Read the model definition and answer for the solid it produces. Units are mm, in the model's axes. Coordinates: 2 decimals unless noted, no trailing zeros. Order: outer loops, then holes, each group sorted by start corner. A loop starts at its lowest first (then second) coordinate and runs counter-clockwise, first axis right, second up. Notation, with made-up numbers: (45, -12.5) -> (62, -12.5) arc R21 cw to (62, 25.5) -> close; hole circle Ø3 at (32, 68.5). An arc over 180 degrees is marked (long way). Answer in a Markdown table with one row per item.
from build123d import *

# Parameters (mm, degrees)
CROQUIS1_R              = 3.25
SALIENTE_EXTRUIR1_DEPTH = 2
CROQUIS2_OUTSIDE_W      = 17.956
CROQUIS2_OUTSIDE_H      = 18.564
CROQUIS2_OUTSIDE_R      = 5
CORTAR_EXTRUIR1_DEPTH   = 1
CORTAR_EXTRUIR1_TAPER   = 45
CHAFL_N2_SIZE           = 0.2
CHAFL_N2_SIZE2          = 0.207106063
CHAFL_N2_PART_2_SIZE    = 0.2
CHAFL_N2_PART_2_SIZE2   = 0.207106063
CHAFL_N2_PART_3_SIZE    = 0.2
CHAFL_N2_PART_3_SIZE2   = 0.207106063
CHAFL_N2_PART_4_SIZE    = 0.2
CHAFL_N2_PART_4_SIZE2   = 0.207106063
CHAFL_N2_PART_5_SIZE    = 0.2
CHAFL_N2_PART_5_SIZE2   = 0.207106063
CHAFL_N2_PART_6_SIZE    = 0.2
CHAFL_N2_PART_6_SIZE2   = 0.207106063


with BuildPart() as part:
    # Croquis1 → Saliente-Extruir1 (new body)
    with BuildSketch(Plane.XY):
        Polygon((-5.395674006, -2.054272462), (-0.918784865, -5.699926991), (4.476889142, -3.645654529), (5.395674006, 2.054272462), (0.918784865, 5.699926991), (-4.476889142, 3.645654529), align=None)
        Circle(CROQUIS1_R, mode=Mode.SUBTRACT)
    extrude(amount=SALIENTE_EXTRUIR1_DEPTH)

    # Croquis2 outside → Cortar-Extruir1 (cut)
    with BuildSketch(Plane(origin=(0, 0, 0), x_dir=(-1, 0, 0), z_dir=(0, 0, -1))):
        Rectangle(CROQUIS2_OUTSIDE_W, CROQUIS2_OUTSIDE_H)
        Circle(CROQUIS2_OUTSIDE_R, mode=Mode.SUBTRACT)
    extrude(amount=-CORTAR_EXTRUIR1_DEPTH, taper=CORTAR_EXTRUIR1_TAPER, mode=Mode.SUBTRACT)

    # Chaflán2
    chafl_n2_edges = [part.edges().sort_by_distance(p)[0] for p in [
        (1.779052139, -4.67279076, 2),
    ]]
    chafl_n2_side = [part.faces().sort_by_distance(p)[0] for p in [
        (1.779052139, -4.67279076, 1.117030845),
    ]]
    chamfer(chafl_n2_edges, length=CHAFL_N2_SIZE, length2=CHAFL_N2_SIZE2, reference=chafl_n2_side[0])

    # Chaflán2 part 2
    chafl_n2_part_2_edges = [part.edges().sort_by_distance(p)[0] for p in [
        (4.936281574, -0.795691033, 2),
    ]]
    chafl_n2_part_2_side = [part.faces().sort_by_distance(p)[0] for p in [
        (4.936281574, -0.795691033, 1.117030845),
    ]]
    chamfer(chafl_n2_part_2_edges, length=CHAFL_N2_PART_2_SIZE, length2=CHAFL_N2_PART_2_SIZE2, reference=chafl_n2_part_2_side[0])

    # Chaflán2 part 3
    chafl_n2_part_3_edges = [part.edges().sort_by_distance(p)[0] for p in [
        (3.157229436, 3.877099727, 2),
    ]]
    chafl_n2_part_3_side = [part.faces().sort_by_distance(p)[0] for p in [
        (3.157229436, 3.877099727, 1.117030845),
    ]]
    chamfer(chafl_n2_part_3_edges, length=CHAFL_N2_PART_3_SIZE, length2=CHAFL_N2_PART_3_SIZE2, reference=chafl_n2_part_3_side[0])

    # Chaflán2 part 4
    chafl_n2_part_4_edges = [part.edges().sort_by_distance(p)[0] for p in [
        (-1.779052139, 4.67279076, 2),
    ]]
    chafl_n2_part_4_side = [part.faces().sort_by_distance(p)[0] for p in [
        (-1.779052139, 4.67279076, 1.117030845),
    ]]
    chamfer(chafl_n2_part_4_edges, length=CHAFL_N2_PART_4_SIZE, length2=CHAFL_N2_PART_4_SIZE2, reference=chafl_n2_part_4_side[0])

    # Chaflán2 part 5
    chafl_n2_part_5_edges = [part.edges().sort_by_distance(p)[0] for p in [
        (-4.936281574, 0.795691033, 2),
    ]]
    chafl_n2_part_5_side = [part.faces().sort_by_distance(p)[0] for p in [
        (-4.936281574, 0.795691033, 1.117030845),
    ]]
    chamfer(chafl_n2_part_5_edges, length=CHAFL_N2_PART_5_SIZE, length2=CHAFL_N2_PART_5_SIZE2, reference=chafl_n2_part_5_side[0])

    # Chaflán2 part 6
    chafl_n2_part_6_edges = [part.edges().sort_by_distance(p)[0] for p in [
        (-3.157229436, -3.877099727, 2),
    ]]
    chafl_n2_part_6_side = [part.faces().sort_by_distance(p)[0] for p in [
        (-3.157229436, -3.877099727, 1.117030845),
    ]]
    chamfer(chafl_n2_part_6_edges, length=CHAFL_N2_PART_6_SIZE, length2=CHAFL_N2_PART_6_SIZE2, reference=chafl_n2_part_6_side[0])


solid = part.part
Q1. The part is cut by section B-B (z = 1.25). Write down the section's boundary in (x, y).
Outcome:
| item | result |
|---|---|
| outline | (-5.4, -2.05) -> (-0.92, -5.7) -> (4.48, -3.65) -> (5.4, 2.05) -> (0.92, 5.7) -> (-4.48, 3.65) -> close; hole circle Ø6.5 at (0, 0) |
Q2. The part is cut by section D-D (z = 0.55). Write down the section's boundary in (x, y).
Outcome:
| item | result |
|---|---|
| outline | (-5.32, -1.58) arc R5.55 ccw to (-5.03, -2.36) -> (-1.29, -5.4) arc R5.55 ccw to (-0.47, -5.53) -> (4.03, -3.82) arc R5.55 ccw to (4.55, -3.17) -> (5.32, 1.58) arc R5.55 ccw to (5.03, 2.36) -> (1.29, 5.4) arc R5.55 ccw to (0.47, 5.53) -> (-4.03, 3.82) arc R5.55 ccw to (-4.55, 3.17) -> close; hole circle Ø6.5 at (0, 0) |
Q3. For a pull along X with two mould halves and no side action, classify faces 1 (the face through (-2.579, -1.978, 0.986)), 2 (the face through (3.19, 3.85, 1.09)), 3 (the face through (-1.741, 4.687, 1.087)) as pulls with the +X half, pulls with the -X half, needs draft (parallel to the pull), parting line crosses it, or undercut.
Outcome:
| item | result |
|---|---|
| face 1 | undercut |
| face 2 | pulls with the +X half |
| face 3 | pulls with the -X half |
Q4. The part is cut by section A-A (x = 0). Write down the section's boundary in (y, z), then the cut area to 3 significant figures.
Outcome:
| item | result |
|---|---|
| outline | (-5.35, 0.35) -> (-5, 0) -> (-3.25, 0) -> (-3.25, 2) -> (-5.13, 2) -> (-5.35, 1.8) -> close; (3.25, 0) -> (5, 0) -> (5.35, 0.35) -> (5.35, 1.8) -> (5.13, 2) -> (3.25, 2) -> close |
| area | 8.23 mm² |
Q5. The part is cut by section C-C (y = 0). Write down the section's boundary in (x, z), then the cut area to 3 significant figures.
Outcome:
| item | result |
|---|---|
| outline | (-5.06, 0.06) -> (-5, 0) -> (-3.25, 0) -> (-3.25, 2) -> (-4.85, 2) -> (-5.06, 1.8) -> close; (3.25, 0) -> (5, 0) -> (5.06, 0.06) -> (5.06, 1.8) -> (4.85, 2) -> (3.25, 2) -> close |
| area | 7.21 mm² |
Q6. Given pin 1 (1.5 mm diameter, centred on x = 1, y = -1, fed in from +Z); pin 2 (1 mm diameter, centred on y = 1.5, z = 1.5, fed in from -X), each flat-ended and moving along its own axis, determine where each tip first touches the part or whether it passes through.
Outcome:
| item | result |
|---|---|
| pin 1 | through |
| pin 2 | x = -4.9 |
Q7. Consider line 1 (Y direction, x = 0, z = 1.15); line 2 (Y direction, x = 0.25, z = 0.6); line 3 (X direction, y = -0.25, z = 0.8). Determine where each line is inside the solid, lowest interval first.
Outcome:
| item | result |
|---|---|
| line 1 | -5.35 to -3.25, 3.25 to 5.35 |
| line 2 | -5.25 to -3.24, 3.24 to 5.45 |
| line 3 | -5.1 to -3.24, 3.24 to 5.02 |
